```python
from build123d import *

# Parameters (mm, degrees)
CYLINDER025_R     = 1
CYLINDER025_DEPTH = 15
CYLINDER022_R     = 2.25
CYLINDER022_DEPTH = 0.9
CYLINDER023_R     = 2.25
CYLINDER023_DEPTH = 0.9
CYLINDER024_R     = 2.25
CYLINDER024_DEPTH = 0.9
CYLINDER021_R     = 2.25
CYLINDER021_DEPTH = 0.9
BOX005_W          = 84.5
BOX005_H          = 50.5
BOX005_DEPTH      = 1.5
BOX004_W          = 80.5
BOX004_H          = 46.5
BOX004_DEPTH      = 1
FILLET001_R       = 1.01


with BuildPart() as hack:
    # Cylinder025 → Cylinder025 (new body)
    with BuildSketch(Plane.XY.offset(-13)):
        Circle(CYLINDER025_R)
    extrude(amount=CYLINDER025_DEPTH)


with BuildPart() as bottom_screw_hole_a:
    # Sketch → Revolution (revolve)
    with BuildSketch(Plane.XZ):
        Polygon((0, 0), (2, 0), (2, 0.2), (1.1, 1.1), (1.1, 3.4), (0, 3.4), align=None)
    revolve(axis=Axis((0, 0, 0), (0, 0, 1)))


with BuildPart() as bottom_screw_hole_a_1:
    # Body placement: moved
    add(bottom_screw_hole_a.part.moved(Location((-37.47, -20.32, 0))))


with BuildPart() as bottom_screw_hole_b:
    # Body001 base: copy of bottom_screw_hole_a
    add(bottom_screw_hole_a_1.part)


with BuildPart() as bottom_screw_hole_b_1:
    # Clone placement: moved
    add(bottom_screw_hole_b.part.moved(Location((37.47, 20.32, 0))))


with BuildPart() as bottom_screw_hole_b_2:
    # Body001 placement: moved
    add(bottom_screw_hole_b_1.part.moved(Location((-37.47, 20.32, 0))))


with BuildPart() as bottom_screw_hole_c:
    # Body002 base: copy of bottom_screw_hole_a
    add(bottom_screw_hole_a_1.part)


with BuildPart() as bottom_screw_hole_c_1:
    # Clone001 placement: moved
    add(bottom_screw_hole_c.part.moved(Location((37.47, 20.32, 0))))


with BuildPart() as bottom_screw_hole_c_2:
    # Body002 placement: moved
    add(bottom_screw_hole_c_1.part.moved(Location((37.47, 20.32, 0))))


with BuildPart() as bottom_screw_hole_d:
    # Body003 base: copy of bottom_screw_hole_a
    add(bottom_screw_hole_a_1.part)


with BuildPart() as bottom_screw_hole_d_1:
    # Clone002 placement: moved
    add(bottom_screw_hole_d.part.moved(Location((37.47, 20.32, 0))))


with BuildPart() as bottom_screw_hole_d_2:
    # Body003 placement: moved
    add(bottom_screw_hole_d_1.part.moved(Location((37.47, -20.32, 0))))


with BuildPart() as bottom_screw_holes:
    # Fusion016 base: copy of bottom_screw_hole_a
    add(bottom_screw_hole_a_1.part)

    # Fusion016: union bottom_screw_hole_b, bottom_screw_hole_c, bottom_screw_hole_d
    add(bottom_screw_hole_b_2.part)
    add(bottom_screw_hole_c_2.part)
    add(bottom_screw_hole_d_2.part)


with BuildPart() as screw_column_b:
    # Cylinder022 → Cylinder022 (new body)
    with BuildSketch(Plane(origin=(-37.47, -20.32, 0), x_dir=(1, 0, 0), z_dir=(0, 0, 1))):
        Circle(CYLINDER022_R)
    extrude(amount=CYLINDER022_DEPTH)


with BuildPart() as screw_column_c:
    # Cylinder023 → Cylinder023 (new body)
    with BuildSketch(Plane(origin=(37.47, 20.32, 0), x_dir=(1, 0, 0), z_dir=(0, 0, 1))):
        Circle(CYLINDER023_R)
    extrude(amount=CYLINDER023_DEPTH)


with BuildPart() as screw_column_d:
    # Cylinder024 → Cylinder024 (new body)
    with BuildSketch(Plane(origin=(37.47, -20.32, 0), x_dir=(1, 0, 0), z_dir=(0, 0, 1))):
        Circle(CYLINDER024_R)
    extrude(amount=CYLINDER024_DEPTH)


with BuildPart() as screw_columns:
    # Cylinder021 → Cylinder021 (new body)
    with BuildSketch(Plane(origin=(-37.47, 20.32, 0), x_dir=(1, 0, 0), z_dir=(0, 0, 1))):
        Circle(CYLINDER021_R)
    extrude(amount=CYLINDER021_DEPTH)

    # Fusion011: union screw_column_b, screw_column_c, screw_column_d
    add(screw_column_b.part)
    add(screw_column_c.part)
    add(screw_column_d.part)


with BuildPart() as screw_columns_1:
    # Fusion011 placement: moved
    add(screw_columns.part.moved(Location((0, 0, 2.5))))


with BuildPart() as external_bottom:
    # Box005 → Box005 (new body)
    with BuildSketch(Plane(origin=(-2, -2, 0), x_dir=(1, 0, 0), z_dir=(0, 0, 1))):
        with Locations((42.25, 25.25)):
            Rectangle(BOX005_W, BOX005_H)
    extrude(amount=BOX005_DEPTH)


with BuildPart() as obj1:
    # Box004 → Box004 (new body)
    with BuildSketch(Plane.XY.offset(1.5)):
        with Locations((40.25, 23.25)):
            Rectangle(BOX004_W, BOX004_H)
    extrude(amount=BOX004_DEPTH)

    # Fusion013: union external_bottom
    add(external_bottom.part)


with BuildPart() as obj1_1:
    # Fusion013 placement: moved
    add(obj1.part.moved(Location((-40.25, -23.25, 0))))

    # Fusion014: union screw_columns
    add(screw_columns_1.part)

    # Cut014: cut bottom_screw_holes
    add(bottom_screw_holes.part, mode=Mode.SUBTRACT)

    # Fillet001
    fillet001_edges = [obj1_1.edges().sort_by_distance(p)[0] for p in [
        (-42.25, -25.25, 0.75),
        (-42.25, 25.25, 0.75),
        (-42.25, 0, 0),
        (0, -25.25, 0),
        (42.25, -25.25, 0.75),
        (0, 25.25, 0),
        (42.25, 25.25, 0.75),
        (42.25, 0, 0),
        (-40.25, -23.25, 2),
        (-40.25, 23.25, 2),
        (40.25, -23.25, 2),
        (40.25, 23.25, 2),
    ]]
    fillet(fillet001_edges, radius=FILLET001_R)


with BuildPart() as obj1_2:
    # Fillet001 placement: moved
    add(obj1_1.part.moved(Location((0, 0, -15))))

    # Fusion017: union hack
    add(hack.part)


solid = obj1_2.part
```
Could you check a few things on this model? Use its own coordinates, in mm. A direction names the side the tool comes from. Give positions to 0.01 mm unless a question says otherwise; leave off trailing zeros. Loops run counter-clockwise (first coordinate to the right, second up) from the corner with the lowest first, then second, coordinate; pieces in that order, holes last. Notation, with made-up numbers: (-32.75, 71.25) - (8.25, 71.25) arc R34 cw to (8.25, 101.25) - close; hole circle Ø3 at (14, 25.25). An arc over 180 degrees is marked (long way). Answer in a Markdown table with one row per item. Add a question column.
Q1. Which directions (+Z, -Z, +X, -X, +Y, -Y) give clear straight access to the entire face, cutting with the end or side of a thin tool? Please do faces 1 (the face through (37.18, 22.55, -12.06)), 2 (the face through (36.6, 19.65, -12.73)).
Q2. If we section it at C-C (y = 0): List the corners of the cut face in (x, z) for me.
Q3. If we section it at D-D (z = -9.25): List the corners of the cut face in (x, y) for me, plus the area to 3 significant figures.
Q4. If we section it at B-B (x = 15): List the corners of the cut face in (y, z) for me.
Q5. If we section it at A-A (x = -37.47): State how many separate pieces and enclosed holes the cut face has, plus the area to 3 significant figures.
Q6. We'd pull the mould along X, two halves only. Please class faces 3 (the face through (-3, -24, -13.5)), 4 (the face through (-36.42, 20.65, -12.73)), 5 (the face through (-36.42, -19.99, -12.73)): +X half, -X half, draft (parallel to the pull), parting line (faces both ways), or undercut.
Q7. For pin 1 (5 mm diameter, centred on x = -38, y = -21.5, fed in from +Z); pin 2 (8 mm diameter, centred on y = -7.5, z = -9, fed in from -X); pin 3 (2 mm diameter, centred on x = 37.47, y = -20.32, fed in from -Z); pin 4 (1.1 mm diameter, centred on x = 9, z = -13, fed in from +Y), each with a flat end and sliding along its axis, tell me the tip position at first contact or that it passes through.
Q8. Please list where these lines run through material, in increasing order: L1, parallel to Y at x = -37.47, z = -12.3; L2, parallel to Y at x = 37.47, z = -13; L3, parallel to Y at x = 37.47, z = -14.9. Write a range as from..to.
The answers:
| question | item | result |
|---|---|---|
| 1 | face 1 | +Z |
| 1 | face 2 | +Z, -Z |
| 2 | outline | (-42.25, -13.99) arc R1.01 ccw to (-41.24, -15) - (41.24, -15) arc R1.01 ccw to (42.25, -13.99) - (42.25, -13.5) - (40.25, -13.5) - (40.25, -12.5) - (1, -12.5) - (1, 2) - (-1, 2) - (-1, -12.5) - (-40.25, -12.5) - (-40.25, -13.5) - (-42.25, -13.5) - close |
| 3 | outline | circle Ø2 at (0, 0) |
| 3 | area | 3.14 mm^2 |
| 4 | outline | (-25.25, -13.99) arc R1.01 ccw to (-24.24, -15) - (24.24, -15) arc R1.01 ccw to (25.25, -13.99) - (25.25, -13.5) - (23.25, -13.5) - (23.25, -12.5) - (-23.25, -12.5) - (-23.25, -13.5) - (-25.25, -13.5) - close |
| 5 | separate pieces | 3 |
| 5 | enclosed holes | 0 |
| 5 | area | 113 mm^2 |
| 6 | face 3 | draft |
| 6 | face 4 | undercut |
| 6 | face 5 | undercut |
| 7 | pin 1 | stops at z = -11.6 |
| 7 | pin 2 | stops at x = -40.25 |
| 7 | pin 3 | passes through |
| 7 | pin 4 | stops at y = 25.25 |
| 8 | L1 | y = -22.57..-21.42, -19.22..-18.07, 18.07..19.22, 21.42..22.57 |
| 8 | L2 | y = -23.25..-21.42, -19.22..19.22, 21.42..23.25 |
| 8 | L3 | y = -24.68..-22.32, -18.32..18.32, 22.32..24.68 |
